```python
from build123d import *

# Parameters (mm, degrees)
SKETCH1_R                          = 36.5125
BOSS_EXTRUDE1_DEPTH                = 1.5875
F_1_4_0_25_DIAMETER_HOLE1_D        = 6.35
F_5_16_0_3125_DIAMETER_HOLE1_D     = 7.9375
F_5_16_0_3125_DIAMETER_HOLE1_DEPTH = 3.302


with BuildPart() as part:
    # Sketch1 → Boss-Extrude1 (new body, symmetric)
    with BuildSketch(Plane.XY):
        Circle(SKETCH1_R)
    extrude(amount=BOSS_EXTRUDE1_DEPTH, both=True)

    # 1/4 (0.25) Diameter Hole1 (through all)
    with Locations(Plane.XY.offset(1.5875)):
        with Locations((-25.4, 0), (25.4, 0)):
            Hole(F_1_4_0_25_DIAMETER_HOLE1_D / 2)

    # 5/16 (0.3125) Diameter Hole1
    with Locations(Plane.XY.offset(1.5875)):
        with Locations((0, 0)):
            Hole(F_5_16_0_3125_DIAMETER_HOLE1_D / 2, depth=F_5_16_0_3125_DIAMETER_HOLE1_DEPTH)


solid = part.part
```
Part model, mm, in its own coordinate system. Round coordinates to 2 decimals unless told otherwise and drop trailing zeros. Write each loop counter-clockwise with the first axis right and the second up, starting at its lowest first coordinate (ties: lowest second). Pieces come first, ordered by that corner, then holes. Notation, with made-up numbers: (14, 48) -> (54, 48) arc R16 cw to (54, 59) -> close; hole circle Ø2 at (61, 22). An arc over 180 degrees is marked (long way). Return JSON: item names as keys, results as strings. Group by question number.
Q1. Saw through at B-B on y = 0. Write the cut outline in (x, z) (1 decimal).
Q2. Saw through at A-A on x = 0. Write the cut outline in (y, z), plus the area to 3 significant figures.
Q3. Mould opens along Y. For faces 1 (the cylindrical face through (22.37, 0.95, -0.02)), 2 (the flat face through (-1, -8, 1.588)), 3 (the cylindrical face through (34.826, 10.967, 0.022)) say: pulls with the +Y half, pulls with the -Y half, needs draft (parallel to the pull), parting line crosses it, or undercut.
Q4. Saw through at D-D on x = 25.4. Write the cut outline in (y, z) (1 decimal), plus the area to 3 significant figures.
Q5. Probe L1, parallel to X at y = -0.5, z = -0.35; L2, parallel to Y at x = -1, z = -0.15; L3, parallel to Y at x = 25.4, z = -0.65 (3 decimals). List the from-to ranges inside material, lowest first. Write a range as [from, to].
Q6. Saw through at C-C on z = 0.3. State how many separate pieces and enclosed holes the cut face has, plus the area to 3 significant figures.
Answer:
{
 "1": {"outline": "(-36.5, -1.6) -> (-28.6, -1.6) -> (-28.6, 1.6) -> (-36.5, 1.6) -> close; (-22.2, -1.6) -> (-4, -1.6) -> (-4, 1.6) -> (-22.2, 1.6) -> close; (4, -1.6) -> (22.2, -1.6) -> (22.2, 1.6) -> (4, 1.6) -> close; (28.6, -1.6) -> (36.5, -1.6) -> (36.5, 1.6) -> (28.6, 1.6) -> close"},
 "2": {"outline": "(-36.51, -1.59) -> (-3.97, -1.59) -> (-3.97, 1.59) -> (-36.51, 1.59) -> close; (3.97, -1.59) -> (36.51, -1.59) -> (36.51, 1.59) -> (3.97, 1.59) -> close", "area": "207 mm2"},
 "3": {"face 1": "undercut", "face 2": "needs draft", "face 3": "parting line crosses it"},
 "4": {"outline": "(-26.2, -1.6) -> (-3.2, -1.6) -> (-3.2, 1.6) -> (-26.2, 1.6) -> close; (3.2, -1.6) -> (26.2, -1.6) -> (26.2, 1.6) -> (3.2, 1.6) -> close", "area": "146 mm2"},
 "5": {"L1": "[-36.51, -28.54], [-22.26, -3.94], [3.94, 22.26], [28.54, 36.51]", "L2": "[-36.5, -3.84], [3.84, 36.5]", "L3": "[-26.23, -3.175], [3.175, 26.23]"},
 "6": {"separate pieces": "1", "enclosed holes": "3", "area": "4,080 mm2"}
}
